Input: part model. Units: mm. Frame: model coordinates. Face numbers are marked on the shaded views. Coordinates: 2 decimals unless noted, no trailing zeros. Order: outer loops, then holes, each group sorted by start corner. A loop starts at its lowest first (then second) coordinate and runs counter-clockwise, first axis right, second up. Notation, with made-up numbers: (46, 13) - (105, 13) arc R28 cw to (105, 38) - close; hole circle Ø9 at (25, -39.5). An arc over 180 degrees is marked (long way). One line per question, with ' | ' between items.
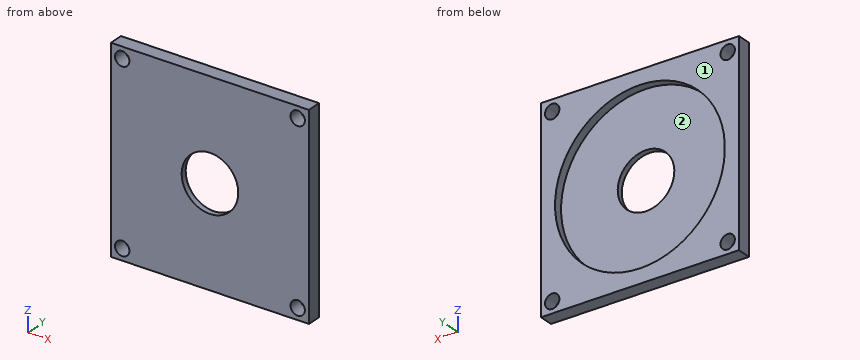
from build123d import *

# Parameters (mm, degrees)
CROQUIS2_W                 = 700
CROQUIS2_H                 = 700
SALIENTE_EXTRUIR1_DEPTH    = 50
CORTAR_EXTRUIR1_DEPTH      = 992.21138008
CORTAR_EXTRUIR1_DEPTH_BACK = 992.21138008
CROQUIS3_R                 = 25.4
CROQUIS4_R                 = 300
CORTAR_EXTRUIR4_DEPTH      = 30
CROQUIS5_R                 = 100
CORTAR_EXTRUIR5_DEPTH      = 20


with BuildPart() as part:
    # Croquis2 → Saliente-Extruir1 (new body)
    with BuildSketch(Plane(origin=(0, 0, 0), x_dir=(1, 0, 0), z_dir=(0, 1, 0))):
        with Locations((350, 350)):
            Rectangle(CROQUIS2_W, CROQUIS2_H)
    extrude(amount=SALIENTE_EXTRUIR1_DEPTH)

    # Croquis3 → Cortar-Extruir1 (cut, two sides: drawn at the far end of the back side and taken through both)
    with BuildSketch(Plane(origin=(0, 50, 0), x_dir=(1, 0, 0), z_dir=(0, 1, 0)).offset(-CORTAR_EXTRUIR1_DEPTH_BACK)):
        with Locations(Location((40, 40, 0), (0, 0, 270))):
            Circle(CROQUIS3_R)
        with Locations(Location((660, 40, 0), (0, 0, 270))):
            Circle(CROQUIS3_R)
        with Locations(Location((660, 660, 0), (0, 0, 270))):
            Circle(CROQUIS3_R)
        with Locations(Location((40, 660, 0), (0, 0, 270))):
            Circle(CROQUIS3_R)
    extrude(amount=CORTAR_EXTRUIR1_DEPTH + CORTAR_EXTRUIR1_DEPTH_BACK, mode=Mode.SUBTRACT)

    # Croquis4 → Cortar-Extruir4 (cut)
    with BuildSketch(Plane(origin=(0, 50, 0), x_dir=(1, 0, 0), z_dir=(0, 1, 0))):
        with Locations(Location((350, 350, 0), (0, 0, 270))):
            Circle(CROQUIS4_R)
    extrude(amount=-CORTAR_EXTRUIR4_DEPTH, mode=Mode.SUBTRACT)

    # Croquis5 → Cortar-Extruir5 (cut)
    with BuildSketch(Plane(origin=(0, 20, 0), x_dir=(1, 0, 0), z_dir=(0, 1, 0))):
        with Locations(Location((350, 350, 0), (0, 0, 270))):
            Circle(CROQUIS5_R)
    extrude(amount=-CORTAR_EXTRUIR5_DEPTH, mode=Mode.SUBTRACT)


solid = part.part
Item 1: Section A-A on x = 350. Return the cut outline in (y, z).
Data:
outline: (0, -700) - (50, -700) - (50, -650) - (20, -650) - (20, -450) - (0, -450) - close; (0, -250) - (20, -250) - (20, -50) - (50, -50) - (50, 0) - (0, 0) - close
Item 2: Section B-B on z = -350. Return the cut outline in (x, y), and give its area (3 significant figures).
Data:
outline: (0, 0) - (250, 0) - (250, 20) - (50, 20) - (50, 50) - (0, 50) - close; (450, 0) - (700, 0) - (700, 50) - (650, 50) - (650, 20) - (450, 20) - close | area: 13,000 mm^2
Item 3: Draft query along Z for the marked faces 1 and 2. Return one class per face: released by +Z, released by -Z, zero draft, split by the parting line, or undercut.
Data:
face 1: zero draft | face 2: undercut
Item 4: Section C-C on z = -660. Return the cut outline in (x, y).
Data:
outline: (0, 0) - (14.6, 0) - (14.6, 50) - (0, 50) - close; (65.4, 0) - (634.6, 0) - (634.6, 50) - (65.4, 50) - close; (685.4, 0) - (700, 0) - (700, 50) - (685.4, 50) - close
Item 5: Section D-D on y = 31.5. Return the cut outline in (x, z).
Data:
outline: (0, -700) - (700, -700) - (700, 0) - (0, 0) - close; hole circle Ø50.8 at (40, -660); hole circle Ø50.8 at (40, -40); hole circle Ø600 at (350, -350); hole circle Ø50.8 at (660, -660); hole circle Ø50.8 at (660, -40)
Item 6: Ray query, line 1 (Z direction, x = 660, y = 35); line 2 (X direction, y = 34, z = -660); line 3 (X direction, y = 31.5, z = -350). Return the intervals inside material, ascending.
Data:
line 1: -700 to -685.4, -634.6 to -65.4, -14.6 to 0 | line 2: 0 to 14.6, 65.4 to 634.6, 685.4 to 700 | line 3: 0 to 50, 650 to 700
Item 7: Contact query for a flat-ended pin moving along its axis: P1, Ø6, axis at x = 230.5, z = -362.5, coming from the +Y side. Output: stop coordinate, or through.
Data:
P1: y = 20
